```python
from build123d import *

# Parameters (mm, degrees)
SKETCH1_W               = 86
SKETCH1_H               = 56
SKETCH1_W_2             = 80
SKETCH1_H_2             = 50
BOSS_EXTRUDE1_DEPTH     = 10
SKETCH2_W               = 86
SKETCH2_H               = 56
BOSS_EXTRUDE2_DEPTH     = 3
SKETCH3_W               = 66
SKETCH3_H               = 36
CUT_EXTRUDE1_DEPTH      = 1
CUT_EXTRUDE1_DEPTH_BACK = 14
SKETCH4_W               = 10
SKETCH4_H               = 10
SKETCH4_R               = 1.5
BOSS_EXTRUDE4_DEPTH     = 13
MIRROR6_COPY_1_SKETCH_W = 10
MIRROR6_COPY_1_SKETCH_H = 10
MIRROR6_COPY_1_SKETCH_R = 1.5
MIRROR6_COPY_1_DEPTH    = 13
SKETCH7_W               = 80.18262614
SKETCH7_H               = 50.033838124
CUT_EXTRUDE3_DEPTH      = 10


with BuildPart() as part:
    # Sketch1 → Boss-Extrude1 (new body)
    with BuildSketch(Plane.XY):
        with Locations((2.183359052, -7.007168459)):
            Rectangle(SKETCH1_W, SKETCH1_H)
        with Locations((2.183359052, -7.007168459)):
            Rectangle(SKETCH1_W_2, SKETCH1_H_2, mode=Mode.SUBTRACT)
    extrude(amount=BOSS_EXTRUDE1_DEPTH)

    # Sketch2 → Boss-Extrude2 (add)
    with BuildSketch(Plane.XY.offset(10)):
        with Locations((2.183359052, -7.007168459)):
            Rectangle(SKETCH2_W, SKETCH2_H)
    extrude(amount=BOSS_EXTRUDE2_DEPTH)

    # Sketch3 → Cut-Extrude1 (cut, two sides)
    with BuildSketch(Plane.XY.offset(13)) as cut_extrude1_sk:
        with Locations((2.183359052, -7.007168459)):
            Rectangle(SKETCH3_W, SKETCH3_H)
    extrude(amount=CUT_EXTRUDE1_DEPTH, mode=Mode.SUBTRACT)
    extrude(cut_extrude1_sk.sketch, amount=-CUT_EXTRUDE1_DEPTH_BACK, mode=Mode.SUBTRACT)

    # Sketch4 → Boss-Extrude4 (add)
    with BuildSketch(Plane.XY.offset(13)):
        with Locations((-40.816640948, -35.007168459)):
            Rectangle(SKETCH4_W, SKETCH4_H)
        with Locations((-43.316640948, -37.507168459)):
            Circle(SKETCH4_R, mode=Mode.SUBTRACT)
    boss_extrude4 = extrude(amount=-BOSS_EXTRUDE4_DEPTH)

    # Mirror5: Boss-Extrude4 across plane
    add(boss_extrude4.mirror(Plane.ZY.offset(-2.183359052)))

    # Mirror6: Boss-Extrude4 across plane
    add(boss_extrude4.mirror(Plane(origin=(0, -7.007168459, 0), x_dir=(0, 0, 1), z_dir=(0, -1, 0))))

    # Mirror6 copy 1 sketch → Mirror6 copy 1 (add)
    with BuildSketch(Plane(origin=(4.366718103, -14.014336918, 13), x_dir=(-1, 0, 0), z_dir=(0, 0, 1))):
        with Locations((-40.816640948, -35.007168459)):
            Rectangle(MIRROR6_COPY_1_SKETCH_W, MIRROR6_COPY_1_SKETCH_H)
        with Locations((-43.316640948, -37.507168459)):
            Circle(MIRROR6_COPY_1_SKETCH_R, mode=Mode.SUBTRACT)
    extrude(amount=-MIRROR6_COPY_1_DEPTH)

    # Sketch7 → Cut-Extrude3 (cut)
    with BuildSketch(Plane(origin=(0, 0, 0), x_dir=(-1, 0, 0), z_dir=(0, 0, -1))):
        with Locations((-2.092045982, -7.024087521)):
            Rectangle(SKETCH7_W, SKETCH7_H)
    extrude(amount=-CUT_EXTRUDE3_DEPTH, mode=Mode.SUBTRACT)


solid = part.part
```
Can you work these out from the model? Positions are in its coordinate system, mm. A direction names the side the tool comes from. Give positions to 0.01 mm unless a question says otherwise; leave off trailing zeros. Order: outer loops, then holes, each group sorted by start corner. A loop starts at its lowest first (then second) coordinate and runs counter-clockwise, first axis right, second up. Notation, with made-up numbers: (38, -39) - (75, -39) arc R6 cw to (75, -28) - close; hole circle Ø3 at (-1, 48.5). An arc over 180 degrees is marked (long way). Use a Markdown table: item, result. Add a question column.
Q1. If we section it at A-A on x = 30: Write out the boundary of the cut face in (y, z), plus the area to 3 significant figures.
Q2. I'm going to push flat-ended pins straight in: pin 1 (1.5 mm diameter, centred on x = 2, z = 11, fed in from +Y); pin 2 (6.5 mm diameter, centred on x = -8, z = 5.5, fed in from -Y); pin 3 (2 mm diameter, centred on y = -24, z = 3, fed in from -X). Where does each tip first touch, or does it pass through?
Q3. On a 3-axis mill with a long thin cutter (end or side, diameter ignored), from which of +Z, -Z, +X, -X, +Y, -Y can I reach the whole of each face in a straight line? I mean faces 1 (the flat face through (-35.817, -38, 7)), 2 (the flat face through (-43, 15.993, 7)), 3 (the flat face through (-37.999, -7, 5)), 4 (the flat face through (2, -25.007, 12)), 5 (the flat face through (-35.817, 24, 7)). Say none if no direction works.
Q4. If we section it at B-B on y = -6: Write out the boundary of the cut face in (x, z), plus the area to 3 significant figures.
Q5. Please list where these lines run through material, in increasing order: line 1 along Y through (x, z) = (24, 9.5); line 2 along X through (y, z) = (-9, 1.25); line 3 along X through (y, z) = (0.5, 11.5).
Q6. If we section it at C-C on y = 13: Write out the boundary of the cut face in (x, z), plus the area to 3 significant figures.
Q7. If we mould it in two halves opening along Y, with no side actions, what happens to faces 6 (the flat face through (-41, 25.993, 7)), 7 (the cylindrical face through (-44.42, -36.49, 6.59)), 8 (the flat face through (-1, 12, 13))? For each: released by +Y, released by -Y, zero draft, split by the parting line, or undercut.
Q8. If we section it at D-D on z = 11: Write out the boundary of the cut face in (x, y), plus the area to 3 significant figures.
Answers follow:
| question | item | result |
|---|---|---|
| 1 | outline | (-35.01, 0) - (-32.04, 0) - (-32.04, 10) - (-25.01, 10) - (-25.01, 13) - (-35.01, 13) - close; (10.99, 10) - (17.99, 10) - (17.99, 0) - (20.99, 0) - (20.99, 13) - (10.99, 13) - close |
| 1 | area | 120 mm^2 |
| 2 | pin 1 | stops at y = 20.99 |
| 2 | pin 2 | stops at y = -35.01 |
| 2 | pin 3 | stops at x = -40.82 |
| 3 | face 1 | +Z, -Z, -Y |
| 3 | face 2 | +Z, -Z, -X |
| 3 | face 3 | -Z |
| 3 | face 4 | +Z, -Z |
| 3 | face 5 | +Z, -Z, +Y |
| 4 | outline | (-40.82, 0) - (-38, 0) - (-38, 10) - (-30.82, 10) - (-30.82, 13) - (-40.82, 13) - close; (35.18, 10) - (42.18, 10) - (42.18, 0) - (45.18, 0) - (45.18, 13) - (35.18, 13) - close |
| 4 | area | 118 mm^2 |
| 5 | line 1 | y = -35.01 to -32.04, 17.99 to 20.99 |
| 5 | line 2 | x = -40.82 to -38, 42.18 to 45.18 |
| 5 | line 3 | x = -40.82 to -30.82, 35.18 to 45.18 |
| 6 | outline | (-40.82, 0) - (-38, 0) - (-38, 10) - (42.18, 10) - (42.18, 0) - (45.18, 0) - (45.18, 13) - (-40.82, 13) - close |
| 6 | area | 316 mm^2 |
| 7 | face 6 | released by +Y |
| 7 | face 7 | undercut |
| 7 | face 8 | zero draft |
| 8 | outline | (-45.82, -40.01) - (-35.82, -40.01) - (-35.82, -35.01) - (40.18, -35.01) - (40.18, -40.01) - (50.18, -40.01) - (50.18, -30.01) - (45.18, -30.01) - (45.18, 15.99) - (50.18, 15.99) - (50.18, 25.99) - (40.18, 25.99) - (40.18, 20.99) - (-35.82, 20.99) - (-35.82, 25.99) - (-45.82, 25.99) - (-45.82, 15.99) - (-40.82, 15.99) - (-40.82, -30.01) - (-45.82, -30.01) - close; hole circle Ø3 at (-43.32, -37.51); hole circle Ø3 at (-43.32, 23.49); hole (-30.82, -25.01) - (35.18, -25.01) - (35.18, 10.99) - (-30.82, 10.99) - close; hole circle Ø3 at (47.68, -37.51); hole circle Ø3 at (47.68, 23.49) |
| 8 | area | 2,710 mm^2 |
